Geometry: final body of the model. Coordinates: model frame, mm. A direction names the side the tool comes from. Round coordinates to 2 decimals unless told otherwise and drop trailing zeros. Loops run counter-clockwise (first coordinate to the right, second up) from the corner with the lowest first, then second, coordinate; pieces in that order, holes last. Notation, with made-up numbers: M 47,8.5 L 78,8.5 A21 ccw 78,28.5 Z; hole C -4.75,-24 d11. An arc over 180 degrees is marked long. Answer as a JSON object with one key per item and string values.
Autodesk Inventor part; units mm, degrees
ref_plane "YZ Plane" through (0, 0, 0) normal (1, 0, 0) x (0, 1, 0)
ref_plane "XZ Plane" through (0, 0, 0) normal (0, 1, 0) x (-1, 0, 0)
ref_plane "XY Plane" through (0, 0, 0) normal (0, 0, 1) x (1, 0, 0)
sketch "Sketch1" plane through (0, 0, 0) normal (0, 0, 1) x (1, 0, 0)
  circle A0 centre (0, 0) radius 180
  circle A1 centre (0, 0) radius 220
  dimension "d0" = 40
  dimension "d1" = 360
extrude "Extrusion1" add sketch "Sketch1" along normal blind 47
sketch "Sketch2" plane through (0, 0, 47) normal (0, 0, 1) x (1, 0, 0)
  circle A0 centre (0, 0) radius 220 construction
  circle A1 centre (0, 0) radius 180 construction
  line L0 (0, 220) -> (0, 180) construction
  circle A2 centre (0, 200) radius 6.25
  dimension "d4" = 12.5
extrude "Extrusion2" cut sketch "Sketch2" against normal through all
sketch "Sketch3" plane through (0, 0, 47) normal (0, 0, 1) x (1, 0, 0)
  circle A0 centre (0, 200) radius 6.25
  circle A1 centre (0, 200) radius 10
  point P0 (0, 0)
  dimension "d10" = 20
extrude "Extrusion3" cut sketch "Sketch3" against normal blind 11
pattern_circular "Circular Pattern1" count 8 over 360 about axis through (0, 0, 0) along (0, 0, 1) of "Extrusion2", "Extrusion3"
sketch "Sketch4" plane through (0, 0, 0) normal (0, 0, -1) x (-1, 0, 0)
  circle A0 centre (0, 0) radius 220
  circle A1 centre (0, 0) radius 225
  dimension "d13" = 5
extrude "Extrusion4" add sketch "Sketch4" against normal blind 10
equation "\"d1\" = Вал_ось_диаметр_КОРМА"
equation "\"d2\" = Барабан_толщина_посад_кольца"
properties part number "ДМС 103 Опорное кольцо вала хвост ПВГ.ipt"
1) Section query D-D (x = -200). Return the cut outline in (y, z), and give its area (3 significant figures).
Results:
{"outline": "M -103.08,0 L -6.25,0 L -6.25,36 L -10,36 L -10,47 L -91.65,47 L -91.65,10 L -103.08,10 Z; M 6.25,0 L 103.08,0 L 103.08,10 L 91.65,10 L 91.65,47 L 10,47 L 10,36 L 6.25,36 Z", "area": "8,170 mm2"}
2) Ray query, line 1 (Y direction, x = 0, z = 38); line 2 (Y direction, x = -139, z = 14); line 3 (X direction, y = 46.5, z = 32.5). Return the intervals inside material, ascending.
Results:
{"line 1": "-220 to -210, -190 to -180, 180 to 190, 210 to 220", "line 2": "-170.53 to -147.18, -135.66 to -114.36, 114.36 to 135.66, 147.18 to 170.53", "line 3": "-215.03 to -173.89, 173.89 to 215.03"}
3) Section query A-A (x = -66.5). Return the cut outline in (y, z), and give its area (3 significant figures).
Results:
{"outline": "M -214.95,0 L -167.27,0 L -167.27,47 L -209.71,47 L -209.71,10 L -214.95,10 Z; M 167.27,0 L 214.95,0 L 214.95,10 L 209.71,10 L 209.71,47 L 167.27,47 Z", "area": "4,090 mm2"}
4) Pull-direction query (X, two-part tool) for faces 3 (the cylindrical face through (-132.986, -136.051, 41.577)), 4 (the cylindrical face through (224.782, 9.893, 4.93)), 5 (the flat face through (68, 168, 0)); classes: +X half, -X half, draft (parallel to the pull), parting line (faces both ways), or undercut.
Results:
{"face 3": "undercut", "face 4": "parting line", "face 5": "draft"}
5) Pin query (flat end, axial travel): P1, Ø5, axis at y = -107.5, z = 30.5, coming from the +X side; P2, Ø11, axis at x = 141.42, y = 141.42, coming from the +Z side; P3, Ø6, axis at x = -2, y = -197, coming from the +Z side; P4, Ø12, axis at x = -169, z = 41.5, coming from the -Y side. Return the tip coordinate at first contact, or that it passes through.
Results:
{"P1": "x = 193.33", "P2": "through", "P3": "z = 36", "P4": "y = -147.75"}
6) Reachability of faces 1 (the cylindrical face through (194.455, -2.884, 18.252)), 2 (the flat face through (135, 142, 36)) from +Z, -Z, +X, -X, +Y, -Y: full face, straight path, thin tool, end or side. Return the list, or none.
Results:
{"face 1": "+Z, -Z", "face 2": "+Z"}
7) Section query C-C (z = 17.5). Count the separate pieces of the cut face and the enclosed holes in it, and give its area (3 significant figures).
Results:
{"separate pieces": "1", "enclosed holes": "9", "area": "49,300 mm2"}
8) Section query B-B (y = 46). Return the cut outline in (x, z).
Results:
{"outline": "M -220.25,0 L -174.02,0 L -174.02,47 L -215.14,47 L -215.14,10 L -220.25,10 Z; M 174.02,0 L 220.25,0 L 220.25,10 L 215.14,10 L 215.14,47 L 174.02,47 Z"}
